Build history of the part. All positions in model axes, mm. Give positions to 0.01 mm unless a question says otherwise; leave off trailing zeros. Put each result on its own line as item: value.
from build123d import *

# Parameters (mm, degrees)
F0_W     = 618
F0_H     = 150
F1_DEPTH = 7
F3_D     = 8.8
F5_D     = 8.8


# Not quite as in the source:
# - a feature names something its author has since deleted; it is built from what else it names


with BuildPart() as f1:
    # F0 (on Front) → F1 (new body)
    with BuildSketch(Plane.XZ):
        with Locations((1, -375)):
            Rectangle(F0_W, F0_H)
    extrude(amount=F1_DEPTH)

    # F3 (through all)
    with Locations(Plane.XZ.offset(7)):
        with Locations((-183, -325), (-133, -325), (185, -325), (185, -425), (135, -425), (-133, -425), (-183, -425), (135, -325)):
            Hole(F3_D / 2)

    # F5 (through all)
    with Locations(Plane.XZ.offset(7)):
        with Locations((-268, -337.5), (-268, -312.5), (270, -337.5), (270, -312.5)):
            Hole(F5_D / 2)


solid = f1.part
1) Wall check: L1, parallel to X at y = -2.5, z = -312.5; L2, parallel to X at y = -5, z = -325; L3, parallel to Z at x = -133, y = -1.5. Give the ranges that are in metal, low to high.
Filled sheet:
L1: -308 to -272.4, -263.6 to 265.6, 274.4 to 310
L2: -308 to -187.4, -178.6 to -137.4, -128.6 to 130.6, 139.4 to 180.6, 189.4 to 310
L3: -450 to -429.4, -420.6 to -329.4, -320.6 to -300
2) Pull direction Y, two halves, no side cores. Call faces 1 (the flat face through (-3, -7, -374)), 2 (the flat face through (-3, 0, -374)): released by +Y, released by -Y, zero draft, split by the parting line, or undercut.
Filled sheet:
face 1: released by -Y
face 2: released by +Y
3) Pin check, flat tip, straight feed: pin 1 (5.5 mm diameter, centred on x = -183, z = -425, fed in from -Y). Stop position of the tip, or through.
Filled sheet:
pin 1: through
